Design review of the part shown in the three views and the two pictorial views. Dimensions are in mm from the part's minimum x, y and z. Give positions to 0.01 mm unless a question says otherwise; leave off trailing zeros. Loops run counter-clockwise (first coordinate to the right, second up) from the corner with the lowest first, then second, coordinate; pieces in that order, holes last.
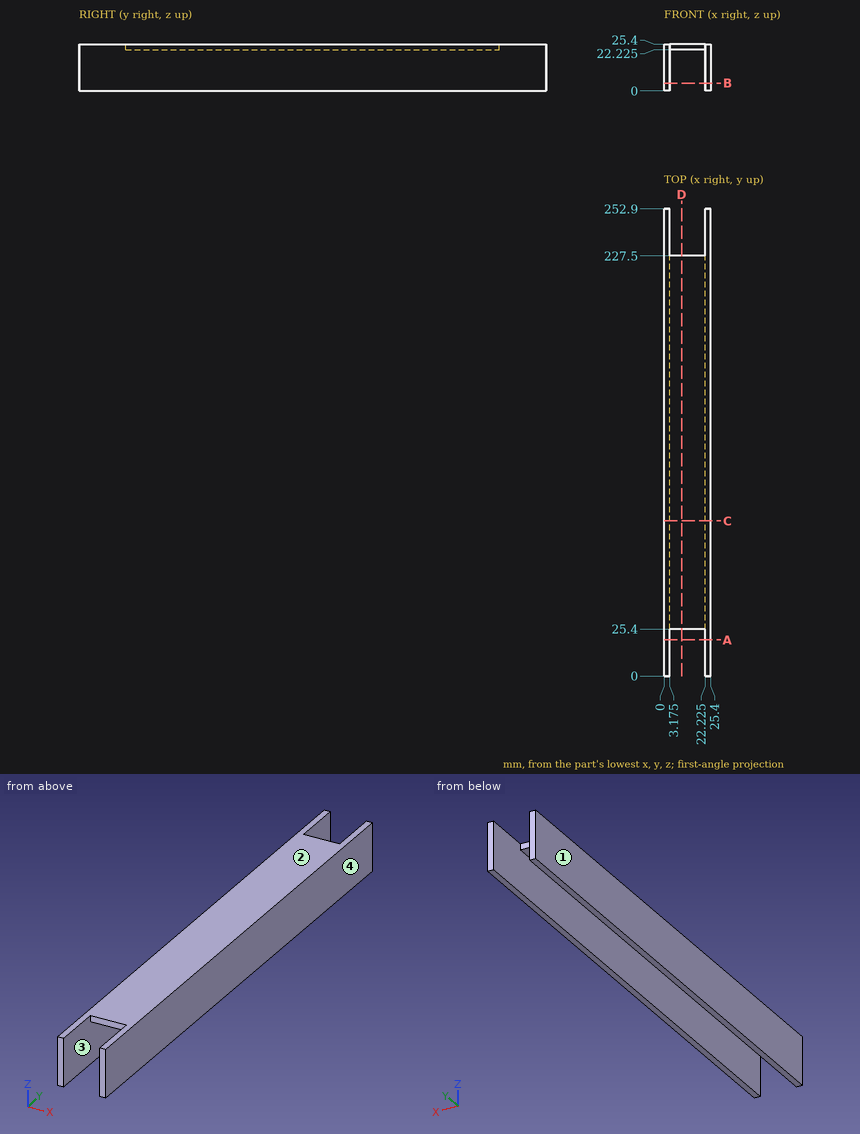
Q1. Mouldability with a two-part tool opening along X and no side actions: class the marked faces 1, 2, 3 and 4 as +X half, -X half, draft (parallel to the pull), parting line (faces both ways), or undercut.
Answers:
face 1: -X half
face 2: draft
face 3: undercut
face 4: +X half
Q2. Consider section A-A on y = 19.5. Give the boundary of the cut face in (x, z) (3 decimals), plus the area to 3 significant figures.
Answers:
outline: (0, 0) - (3.175, 0) - (3.175, 25.4) - (0, 25.4) - close; (22.225, 0) - (25.4, 0) - (25.4, 25.4) - (22.225, 25.4) - close
area: 161 mm2
Q3. Consider section D-D on x = 9.5. Give the boundary of the cut face in (y, z) (3 decimals), plus the area to 3 significant figures.
Answers:
outline: (25.4, 22.225) - (227.5, 22.225) - (227.5, 25.4) - (25.4, 25.4) - close
area: 642 mm2
Q4. Consider section B-B on z = 4.25. Give the boundary of the cut face in (x, y) (3 decimals).
Answers:
outline: (0, 0) - (3.175, 0) - (3.175, 252.9) - (0, 252.9) - close; (22.225, 0) - (25.4, 0) - (25.4, 252.9) - (22.225, 252.9) - close
Q5. Consider section C-C on y = 84. Give the boundary of the cut face in (x, z) (3 decimals).
Answers:
outline: (0, 0) - (3.175, 0) - (3.175, 22.225) - (22.225, 22.225) - (22.225, 0) - (25.4, 0) - (25.4, 25.4) - (0, 25.4) - close
Q6. For probe 1 along X at (y, z) = (75.5, 17.75) (3 decimals); probe 2 along Z at (x, y) = (18.25, 140) (3 decimals); probe 3 along Y at (x, z) = (4, 23.75), list the stretches that pass through material, from the lowest coordinate up.
Answers:
probe 1: x = 0 to 3.175, 22.225 to 25.4
probe 2: z = 22.225 to 25.4
probe 3: y = 25.4 to 227.5
Q7. For pin 1 Ø12 at (x, y) = (14, 184) entering from -Z (3 decimals); pin 2 Ø1 at (x, z) = (17, 23.5) entering from -Y; pin 3 Ø1.6 at (x, z) = (9, 23.5) entering from +Y, all flat-tipped, find the tip position at first contact; note any pin that passes through.
Answers:
pin 1: stops at z = 22.225
pin 2: stops at y = 25.4
pin 3: stops at y = 227.5
